from build123d import *

# Parameters (mm, degrees)
BOSS_EXTRUDE1_DEPTH  = 2
BOSS_EXTRUDE6_DEPTH  = 4.5
CUT_EXTRUDE6_DEPTH   = 4.5
BOSS_EXTRUDE14_DEPTH = 2.3
SKETCH32_R           = 2.1
CUT_EXTRUDE7_DEPTH   = 2.3
SKETCH33_W           = 12.5
SKETCH33_H           = 1.343145751
BOSS_EXTRUDE15_DEPTH = 1.2
SKETCH35_W           = 5.479645997
SKETCH35_H           = 5.327993755
CUT_EXTRUDE8_DEPTH   = 2.4
SKETCH36_W           = 3.7
SKETCH36_H           = 1.827993755
CUT_EXTRUDE9_DEPTH   = 2.4
SKETCH37_R           = 3.9
BOSS_EXTRUDE16_DEPTH = 4.4
CUT_EXTRUDE10_DEPTH  = 7.4
SKETCH43_R           = 2.5
BOSS_EXTRUDE17_DEPTH = 1.2
SKETCH44_R           = 0.95
CUT_EXTRUDE11_DEPTH  = 11
SKETCH45_R           = 2
CUT_EXTRUDE12_DEPTH  = 4.5
SKETCH52_R           = 0.75
CUT_EXTRUDE13_DEPTH  = 10


with BuildPart() as part:
    # Sketch3 → Boss-Extrude1 (new body)
    with BuildSketch(Plane.XY):
        with BuildLine():
            Line((8, 0), (9, -2.5))
            Line((9, -2.5), (9, -7))
            Line((9, -7), (21.5, -7))
            Line((21.5, -7), (25.050252532, -4.949747468))
            ThreePointArc((25.050252532, -4.949747468), (36.467156728, -2.678784027), (30, 7))
            Line((30, 7), (27, 7.5))
            Line((27, 7.5), (5.656854249, 7.5))
            Line((5.656854249, 7.5), (5.656854249, 5.656854249))
            ThreePointArc((5.656854249, 5.656854249), (7.39103626, 3.061467459), (8, 0))
        make_face()
    extrude(amount=BOSS_EXTRUDE1_DEPTH)

    # Sketch22 → Boss-Extrude6 (add)
    with BuildSketch(Plane.XY.offset(2)):
        with BuildLine():
            Line((5.656854249, 5.656854249), (2.486790148, 5.656854249))
            Line((2.486790148, 5.656854249), (2.486790148, 7.5))
            Line((2.486790148, 7.5), (5.656854249, 7.5))
            Line((5.656854249, 7.5), (21.5, 7.5))
            Line((21.5, 7.5), (27, 7.5))
            Line((27, 7.5), (27, 2.172006245))
            Line((27, 2.172006245), (23.275126266, 2.172006245))
            Line((23.275126266, 2.172006245), (23.275126266, -5.974873734))
            Line((23.275126266, -5.974873734), (21.5, -7))
            Line((21.5, -7), (9, -7))
            Line((9, -7), (9, -2.5))
            Line((9, -2.5), (8, 0))
            ThreePointArc((8, 0), (7.39103626, 3.061467459), (5.656854249, 5.656854249))
        make_face()
    extrude(amount=BOSS_EXTRUDE6_DEPTH)

    # Sketch26 → Cut-Extrude6 (cut)
    with BuildSketch(Plane.XY.offset(2)):
        Polygon((18.098080448, 5.3), (2.530052458, 5.3), (2.530052458, 4), (18.098080448, 4), (27, 4), (27, 5.3), align=None)
    extrude(amount=CUT_EXTRUDE6_DEPTH, mode=Mode.SUBTRACT)


with BuildPart() as body_2:
    # Sketch31 → Boss-Extrude14 (new body)
    with BuildSketch(Plane.XY.offset(6.5)):
        with BuildLine():
            Line((2.432688066, 5.656854249), (0, 5.656854249))
            ThreePointArc((0, 5.656854249), (-5.656854249, 0), (0, -5.656854249))
            Line((0, -5.656854249), (9, -5.656854249))
            Line((9, -5.656854249), (9, -7))
            Line((9, -7), (21.5, -7))
            Line((21.5, -7), (23.275126266, -5.974873734))
            Line((23.275126266, -5.974873734), (23.275126266, 2.172006245))
            Line((23.275126266, 2.172006245), (27, 2.172006245))
            Line((27, 2.172006245), (27, 7.5))
            Line((27, 7.5), (2.486790148, 7.5))
            Line((2.486790148, 7.5), (2.432688066, 5.656854249))
        make_face()
    extrude(amount=BOSS_EXTRUDE14_DEPTH)

    # Sketch32 → Cut-Extrude7 (cut)
    with BuildSketch(Plane.XY.offset(8.8)):
        Circle(SKETCH32_R)
    extrude(amount=-CUT_EXTRUDE7_DEPTH, mode=Mode.SUBTRACT)

    # Sketch33 → Boss-Extrude15 (add)
    with BuildSketch(Plane.XY.offset(8.8)):
        with Locations((15.25, -6.328427125)):
            Rectangle(SKETCH33_W, SKETCH33_H)
        Polygon((2.486790148, 7.5), (21.5, 7.5), (21.5, 5.656854249), (2.432688066, 5.656854249), align=None)
    extrude(amount=BOSS_EXTRUDE15_DEPTH)


with BuildPart() as cut_extrude8_tool:
    # Sketch35 → Cut-Extrude8 (new body)
    with BuildSketch(Plane.XY.offset(8.8)):
        with Locations((24.260177002, 4.836003123)):
            Rectangle(SKETCH35_W, SKETCH35_H)
    extrude(amount=-CUT_EXTRUDE8_DEPTH)


with BuildPart() as part_1:
    add(part.part)

    # Cut-Extrude8: cut by cut_extrude8_tool
    add(cut_extrude8_tool.part, mode=Mode.SUBTRACT)

    # Sketch36 → Cut-Extrude9 (cut)
    with BuildSketch(Plane.XY.offset(6.4)):
        with Locations((25.15, 3.086003123)):
            Rectangle(SKETCH36_W, SKETCH36_H)
    extrude(amount=-CUT_EXTRUDE9_DEPTH, mode=Mode.SUBTRACT)

    # Sketch37 → Boss-Extrude16 (add)
    with BuildSketch(Plane.XY.offset(2)):
        with Locations((30, 0)):
            Circle(SKETCH37_R)
    extrude(amount=BOSS_EXTRUDE16_DEPTH)

    # Sketch39 → Cut-Extrude10 (cut, through all)
    with BuildSketch(Plane.XY.offset(6.4)):
        with BuildLine():
            Line((29, 1.732050808), (29, -1.732050808))
            ThreePointArc((29, -1.732050808), (32, 0), (29, 1.732050808))
        make_face()
    extrude(amount=-CUT_EXTRUDE10_DEPTH, mode=Mode.SUBTRACT)


with BuildPart() as body_2_1:
    add(body_2.part)

    # Cut-Extrude8: cut by cut_extrude8_tool
    add(cut_extrude8_tool.part, mode=Mode.SUBTRACT)

    # Sketch43 → Boss-Extrude17 (add)
    with BuildSketch(Plane.XY.offset(8.8)):
        with Locations((11.5, 0)):
            Circle(SKETCH43_R)
        with Locations((18, 0)):
            Circle(SKETCH43_R)
    extrude(amount=BOSS_EXTRUDE17_DEPTH)


with BuildPart() as cut_extrude11_tool:
    # Sketch44 → Cut-Extrude11 (new body, through all)
    with BuildSketch(Plane.XY.offset(10)):
        with Locations((11.5, 0)):
            Circle(SKETCH44_R)
        with Locations((18, 0)):
            Circle(SKETCH44_R)
    extrude(amount=-CUT_EXTRUDE11_DEPTH)


with BuildPart() as part_2:
    add(part_1.part)

    # Cut-Extrude11: cut by cut_extrude11_tool
    add(cut_extrude11_tool.part, mode=Mode.SUBTRACT)

    # Sketch45 → Cut-Extrude12 (cut)
    with BuildSketch(Plane(origin=(0, 0, 0), x_dir=(-1, 0, 0), z_dir=(0, 0, -1))):
        with Locations((-11.5, 0)):
            Circle(SKETCH45_R)
        with Locations((-18, 0)):
            Circle(SKETCH45_R)
    extrude(amount=-CUT_EXTRUDE12_DEPTH, mode=Mode.SUBTRACT)


with BuildPart() as body_2_2:
    add(body_2_1.part)

    # Cut-Extrude11: cut by cut_extrude11_tool
    add(cut_extrude11_tool.part, mode=Mode.SUBTRACT)

    # Sketch52 → Cut-Extrude13 (cut, along a direction that is not the sketch's normal)
    with BuildSketch(Plane.XZ.offset(-5.656854249)):
        with Locations((18.235476819, 10)):
            Circle(SKETCH52_R)
    extrude(amount=-CUT_EXTRUDE13_DEPTH, dir=(0.640410196, -0.76803306, 0), mode=Mode.SUBTRACT)


solid = part_2.part
Geometry check sheet. Reference: the model listing, model coordinates, mm. A direction names the side the tool comes from. Round coordinates to 2 decimals unless told otherwise and drop trailing zeros. Loops run counter-clockwise (first coordinate to the right, second up) from the corner with the lowest first, then second, coordinate; pieces in that order, holes last.
Item 1: Thickness scan on line 1 (Y direction, x = 18, z = 3.45); line 2 (Y direction, x = 18, z = 5.35); line 3 (Y direction, x = 11.5, z = 1.6). Record the ranges inside material, lowest first.
Item 2: Mould release check, pull along X, two halves, no side actions. Record for faces 1 (the cylindrical face through (7.41, 3.02, 3.2)), 2 (the flat face through (23.3, 3, 5)), 3 (the flat face through (28, 0, 6.4)): pulls with the +X half, pulls with the -X half, needs draft (parallel to the pull), parting line crosses it, or undercut.
Item 3: Cross-section at D-D on x = 22. Record the boundary of the cut face in (y, z).
Item 4: Cross-section at C-C on x = 18. Record the boundary of the cut face in (y, z).
Item 5: Access from +Z, -Z, +X, -X, +Y, -Y to the whole of each face (thin tool, end or side, straight path). Record for faces 4 (the flat face through (25, 2.172, 3)), 5 (the flat face through (4, 7, 2)), 6 (the flat face through (4, 5.657, 4)), 7 (the flat face through (29, 0, 3)), 8 (the flat face through (23.275, -2, 4)).
Item 6: Cross-section at A-A on z = 3. Record the boundary of the cut face in (x, y), then the cut area to 3 significant figures.
Item 7: Gauge pin test, flat ends, axial feed: pin 1 (0.9 mm diameter, centred on x = 25, y = 3, fed in from +Z); pin 2 (3 mm diameter, centred on x = 30, y = 0, fed in from +Z); pin 3 (1.7 mm diameter, centred on y = 0, z = 4.5, fed in from +X); pin 4 (1.1 mm diameter, centred on x = 18, y = 0, fed in from +Z). Record the tip position at first contact, or that the pin passes through.
Item 8: Cross-section at B-B on y = 0.5. Count the separate pieces of the cut face and the enclosed holes in it, then the cut area to 3 significant figures.
Answer sheet:
1. line 1: y = -7 to -2, 2 to 4, 5.3 to 7.5
1. line 2: y = -7 to -0.95, 0.95 to 4, 5.3 to 7.5
1. line 3: y = -7 to -2, 2 to 7.5
2. face 1: pulls with the -X half
2. face 2: undercut
2. face 3: needs draft
3. outline: (-6.71, 0) - (7.5, 0) - (7.5, 6.4) - (5.3, 6.4) - (5.3, 2) - (4, 2) - (4, 6.4) - (2.17, 6.4) - (2.17, 6.5) - (-6.71, 6.5) - close
4. outline: (-7, 0) - (-2, 0) - (-2, 4.5) - (-0.95, 4.5) - (-0.95, 6.5) - (-7, 6.5) - close; (0.95, 4.5) - (2, 4.5) - (2, 0) - (7.5, 0) - (7.5, 6.5) - (5.3, 6.5) - (5.3, 2) - (4, 2) - (4, 6.5) - (0.95, 6.5) - close
5. face 4: +Z
5. face 5: -Z, -X, +Y, -Y
5. face 6: +Z, -Z, -X, -Y
5. face 7: +Z, -Z
5. face 8: +Z, -Y
6. outline: (2.49, 5.66) - (5.66, 5.66) arc R8 cw to (5.99, 5.3) - (27, 5.3) - (27, 7.5) - (2.49, 7.5) - close; (6.93, 4) arc R8 cw to (8, 0) - (9, -2.5) - (9, -7) - (21.5, -7) - (23.28, -5.97) - (23.28, 2.17) - (26.76, 2.17) arc R3.9 ccw (long way) to (27, 2.49) - (27, 4) - close; hole circle Ø4 at (11.5, 0); hole circle Ø4 at (18, 0); hole (29, -1.73) arc R2 ccw (long way) to (29, 1.73) - close
6. area: 235 mm2
7. pin 1: stops at z = 4
7. pin 2: stops at z = 6.4
7. pin 3: stops at x = 33.9
7. pin 4: passes through
8. separate pieces: 4
8. enclosed holes: 0
8. area: 101 mm2
